Source: three-view drawing plus pictorial views. Frame: mm from the lowest corner of the part. A direction names the side the tool comes from. Round coordinates to 2 decimals unless told otherwise and drop trailing zeros. Loops run counter-clockwise (first coordinate to the right, second up) from the corner with the lowest first, then second, coordinate; pieces in that order, holes last. Notation, with made-up numbers: (38, -13.5) -> (61, -13.5) arc R8 ccw to (61, -6.5) -> close; hole circle Ø2 at (70.25, -20.5). An arc over 180 degrees is marked (long way). Answer as a JSON object with one key per item and string values. Group by question number.
Item 1: Section query D-D on x = 44. Return loops of the section in (y, z), and give its area (3 significant figures).
Item 2: Draft query along Z for the marked faces 1, 2, 3 and 4. Return one class per face: released by +Z, released by -Z, zero draft, split by the parting line, or undercut.
Item 3: Section query C-C on x = 19.5. Return loops of the section in (y, z).
Item 4: Set-up query: the marked faces 5, 6, 7, 8 and 9. Return all of +Z, -Z, +X, -X, +Y, -Y with unobstructed straight access to the full face (end or side cutting, diameter ignored); none if empty.
Item 5: Pin query (flat end, axial travel): pin 1 (3 mm diameter, centred on x = 34, y = 3, fed in from -Z). Return the tip coordinate at first contact, or that it passes through.
Item 6: Material intervals for line 1 (Z direction, x = 29.5, y = 2.75); line 2 (X direction, y = 0.75, z = 24.5) (1 decimal); line 3 (X direction, y = 4.25, z = 47.5) (1 decimal), sorted ascending. Write a range as [from, to].
Item 7: Section query B-B on x = 58. Return loops of the section in (y, z).
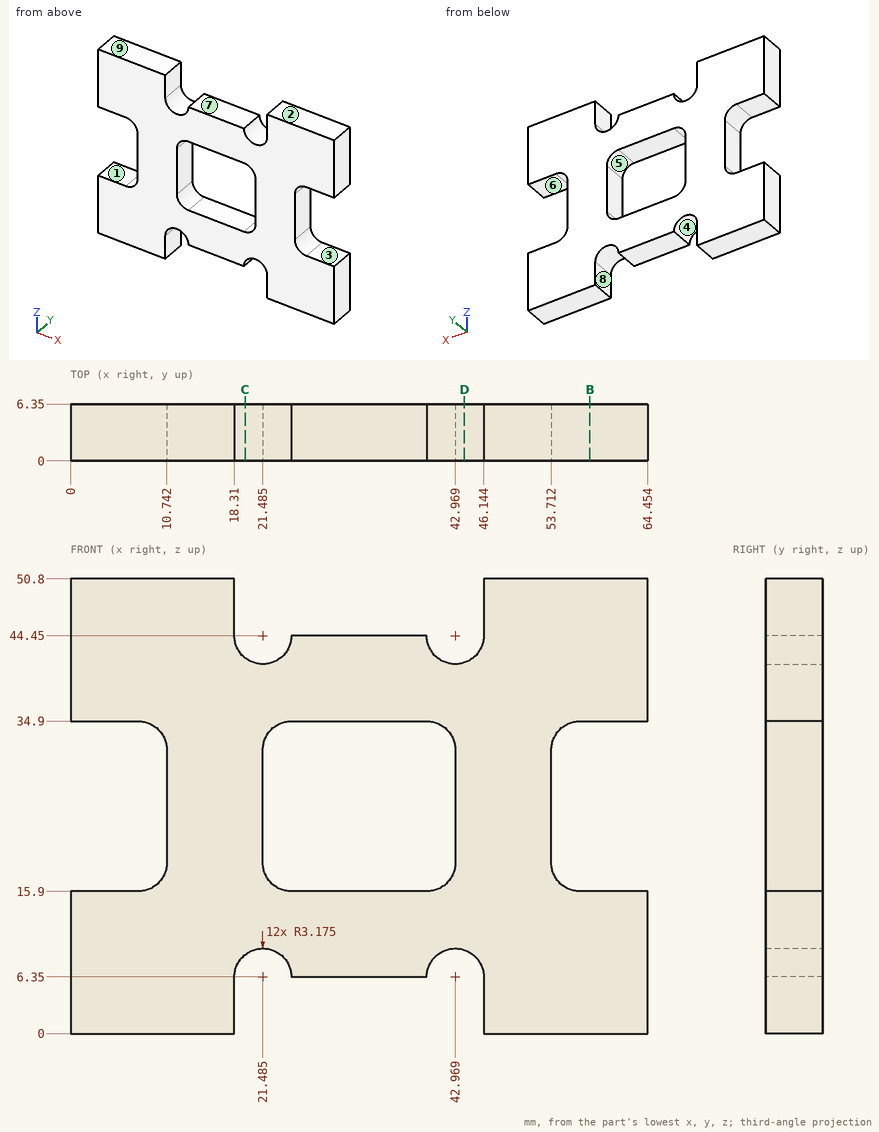
Solved:
{
 "1": {"outline": "(0, 9.35) -> (6.35, 9.35) -> (6.35, 41.45) -> (0, 41.45) -> close", "area": "204 mm²"},
 "2": {"face 1": "undercut", "face 2": "released by +Z", "face 3": "undercut", "face 4": "released by -Z"},
 "3": {"outline": "(0, 8.83) -> (6.35, 8.83) -> (6.35, 41.97) -> (0, 41.97) -> close"},
 "4": {"face 5": "+Y, -Y", "face 6": "+X, +Y, -Y", "face 7": "+Z, +Y, -Y", "face 8": "-Z, +Y, -Y", "face 9": "+Z, +X, -X, +Y, -Y"},
 "5": {"pin 1": "z = 6.35"},
 "6": {"line 1": "[6.35, 15.9], [34.9, 44.45]", "line 2": "[10.7, 21.5], [43, 53.7]", "line 3": "[0, 18.3], [46.1, 64.5]"},
 "7": {"outline": "(0, 0) -> (6.35, 0) -> (6.35, 15.9) -> (0, 15.9) -> close; (0, 34.9) -> (6.35, 34.9) -> (6.35, 50.8) -> (0, 50.8) -> close"}
}
